Design review of the part built by this model. Coordinates are the model's own, in mm. Give positions to 0.01 mm unless a question says otherwise; leave off trailing zeros. Write each loop counter-clockwise with the first axis right and the second up, starting at its lowest first coordinate (ties: lowest second). Pieces come first, ordered by that corner, then holes. Notation, with made-up numbers: (79.5, 61) -> (123.5, 61) arc R20 ccw to (123.5, 92) -> close; hole circle Ø11 at (-11.75, 84). An arc over 180 degrees is marked (long way). Answer as a JSON object with one key per item and string values.
```python
from build123d import *

# Parameters (mm, degrees)
MODEL_R                 = 1.5
SALIENTE_EXTRUIR1_DEPTH = 3


with BuildPart() as part:
    # Model → Saliente-Extruir1 (new body)
    with BuildSketch(Plane.XY):
        with BuildLine():
            Line((174.227054575, 213.178720063), (174.227054575, 204.178720063))
            ThreePointArc((174.227054575, 204.178720063), (174.569596678, 202.456644617), (175.545074059, 200.996739548))
            Line((175.545074059, 200.996739548), (184.545074059, 191.996739548))
            ThreePointArc((184.545074059, 191.996739548), (187.727054575, 190.678720063), (190.90903509, 191.996739548))
            Line((190.90903509, 191.996739548), (199.90903509, 200.996739548))
            ThreePointArc((199.90903509, 200.996739548), (200.884512471, 202.456644617), (201.227054575, 204.178720063))
            Line((201.227054575, 204.178720063), (201.227054575, 226.678720063))
            Line((201.227054575, 226.678720063), (174.227054575, 226.678720063))
            Line((174.227054575, 226.678720063), (174.227054575, 213.178720063))
        make_face()
        with Locations((187.727054575, 204.178720063)):
            Circle(MODEL_R, mode=Mode.SUBTRACT)
        with Locations((178.727054575, 204.178720063)):
            Circle(MODEL_R, mode=Mode.SUBTRACT)
        with Locations((187.727054575, 213.178720063)):
            Circle(MODEL_R, mode=Mode.SUBTRACT)
        with Locations((178.727054575, 213.178720063)):
            Circle(MODEL_R, mode=Mode.SUBTRACT)
        with Locations((196.727054575, 213.178720063)):
            Circle(MODEL_R, mode=Mode.SUBTRACT)
        with Locations((187.727054575, 195.178720063)):
            Circle(MODEL_R, mode=Mode.SUBTRACT)
        with Locations((196.727054575, 204.178720063)):
            Circle(MODEL_R, mode=Mode.SUBTRACT)
        with Locations((187.727054575, 222.178720063)):
            Circle(MODEL_R, mode=Mode.SUBTRACT)
        with Locations((178.727054575, 222.178720063)):
            Circle(MODEL_R, mode=Mode.SUBTRACT)
        with Locations((196.727054575, 222.178720063)):
            Circle(MODEL_R, mode=Mode.SUBTRACT)
    extrude(amount=SALIENTE_EXTRUIR1_DEPTH)


solid = part.part
```
(1) For line 1 along X through (y, z) = (204.5, 1.35); line 2 along X through (y, z) = (213, 1.65); line 3 along Y through (x, z) = (197.25, 1.35), list the stretches that pass through material, from the lowest coordinate up.
Here are the results:
{"line 1": "x = 174.23 to 177.26, 180.19 to 186.26, 189.19 to 195.26, 198.19 to 201.23", "line 2": "x = 174.23 to 177.24, 180.22 to 186.24, 189.22 to 195.24, 198.22 to 201.23", "line 3": "y = 198.34 to 202.77, 205.58 to 211.77, 214.58 to 220.77, 223.58 to 226.68"}
(2) We need section C-C, the plane z = 1.3. Give the number of separate pieces and of enclosed holes in the cut face, then the cut area to 3 significant figures.
Here are the results:
{"separate pieces": "1", "enclosed holes": "10", "area": "764 mm²"}
(3) We need section A-A, the plane x = 187.5. State the section outline as (y, z) points, then the cut area to 3 significant figures.
Here are the results:
{"outline": "(190.68, 0) -> (193.7, 0) -> (193.7, 3) -> (190.68, 3) -> close; (196.66, 0) -> (202.7, 0) -> (202.7, 3) -> (196.66, 3) -> close; (205.66, 0) -> (211.7, 0) -> (211.7, 3) -> (205.66, 3) -> close; (214.66, 0) -> (220.7, 0) -> (220.7, 3) -> (214.66, 3) -> close; (223.66, 0) -> (226.68, 0) -> (226.68, 3) -> (223.66, 3) -> close", "area": "72.4 mm²"}
(4) We need section D-D, the plane x = 196.25. State the section outline as (y, z) points.
Here are the results:
{"outline": "(197.34, 0) -> (202.76, 0) -> (202.76, 3) -> (197.34, 3) -> close; (205.6, 0) -> (211.76, 0) -> (211.76, 3) -> (205.6, 3) -> close; (214.6, 0) -> (220.76, 0) -> (220.76, 3) -> (214.6, 3) -> close; (223.6, 0) -> (226.68, 0) -> (226.68, 3) -> (223.6, 3) -> close"}
(5) Clearance check with a flat-ended pin moving along its axis: pin 1 (1.8 mm diameter, centred on x = 178.73, y = 222.18, fed in from +Z). State where the tip first meets the part, or that it passes through.
Here are the results:
{"pin 1": "passes through"}
(6) The part is to be moulded in two halves that separate along Y. For faces 1 (the flat face through (188, 209, 0)), 2 (the cylindrical face through (189.158, 204.629, 1.479)), 3 (the cylindrical face through (174.56, 202.48, 1.48)), say which applies: +Y half, -Y half, draft (parallel to the pull), parting line (faces both ways), or undercut.
Here are the results:
{"face 1": "draft", "face 2": "undercut", "face 3": "-Y half"}
(7) We need section B-B, the plane x = 179. State the section outline as (y, z) points.
Here are the results:
{"outline": "(197.54, 0) -> (202.7, 0) -> (202.7, 3) -> (197.54, 3) -> close; (205.65, 0) -> (211.7, 0) -> (211.7, 3) -> (205.65, 3) -> close; (214.65, 0) -> (220.7, 0) -> (220.7, 3) -> (214.65, 3) -> close; (223.65, 0) -> (226.68, 0) -> (226.68, 3) -> (223.65, 3) -> close"}
